Here's how the part is built. I have some questions about the finished solid (model axes, mm). Face numbers are marked on the shaded views. A direction names the side the tool comes from. Give positions to 0.01 mm unless a question says otherwise; leave off trailing zeros. Loops run counter-clockwise (first coordinate to the right, second up) from the corner with the lowest first, then second, coordinate; pieces in that order, holes last.
Q1. For the marked faces 4, 5 and 6, which set-ups out of +Z, -Z, +X, -X, +Y, -Y let a thin tool reach every point of the face, with its end or its side?
Q2. I need wall thicknesses on probe 1 along X at (y, z) = (14.5, 7.5); probe 2 along X at (y, z) = (4, 7); probe 3 along Y at (x, z) = (2, -16.5). Which ranges of each line are inside material? Lowest first, please.
Q3. Suppose I cut it at C-C (y = 13.5). List the corners of the cut face in (x, z) for me, and give its area (3 significant figures).
Q4. Suppose I cut it at B-B (z = 0). List the corners of the cut face in (x, y) for me, and give its area (3 significant figures).
Q5. Suppose I cut it at D-D (y = 6.5). List the corners of the cut face in (x, z) for me.
Q6. Suppose I cut it at A-A (x = 0). List the corners of the cut face in (y, z) for me, and give its area (3 significant figures).
Q7. Thinking about a two-plate mould opening in X: for the marked faces 1, 2 and 3, which applies, pulls with the +X half, pulls with the -X half, needs draft (parallel to the pull), parting line crosses it, or undercut?
Q8. I'm going to push flat-ended pins straight in: P1, Ø2, axis at x = -1, z = 21.5, coming from the -Y side; P2, Ø6.5, axis at x = -12.99, z = 7.5, coming from the -Y side; P3, Ø1, axis at x = 15.5, z = -16, coming from the +Y side; P4, Ø1, axis at x = -15, y = 10, coming from the -Z side. Where does each tip first touch, or does it pass through?
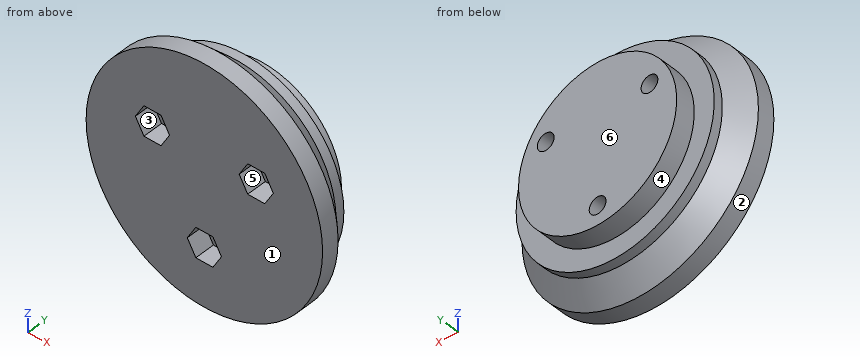
```python
from build123d import *

# Parameters (mm, degrees)
CUT_EXTRUDE1_REACH = 46.995
SKETCH2_R          = 2.1
CUT_EXTRUDE2_DEPTH = 5


with BuildPart() as part:
    # Sketch1 → Revolve1 (revolve)
    with BuildSketch(Plane.XY):
        Polygon((0, 16.5), (19.8, 16.5), (19.8, 11.5), (24.8, 11.5), (24.8, 9.2), (29.6, 4.4), (29.6, 0), (0, 0), align=None)
    revolve(axis=Axis((0, 0, 0), (0, 1, 0)))

    # Sketch2 → Cut-Extrude1 (cut, up to next)
    with BuildSketch(Plane(origin=(0, 16.5, 0), x_dir=(1, 0, 0), z_dir=(0, 1, 0)), mode=Mode.PRIVATE) as cut_extrude1_sk1:
        with Locations(Location((0, 15, 0), (0, 0, 270))):
            Circle(SKETCH2_R)
    cut_extrude1_tool1 = extrude(cut_extrude1_sk1.sketch, amount=-CUT_EXTRUDE1_REACH, mode=Mode.PRIVATE) & part.part
    # Sketch2 → Cut-Extrude1 (cut, up to next)
    with BuildSketch(Plane(origin=(0, 16.5, 0), x_dir=(1, 0, 0), z_dir=(0, 1, 0)), mode=Mode.PRIVATE) as cut_extrude1_sk2:
        with Locations(Location((-12.990381057, -7.5, 0), (0, 0, 270))):
            Circle(SKETCH2_R)
    cut_extrude1_tool2 = extrude(cut_extrude1_sk2.sketch, amount=-CUT_EXTRUDE1_REACH, mode=Mode.PRIVATE) & part.part
    # Sketch2 → Cut-Extrude1 (cut, up to next)
    with BuildSketch(Plane(origin=(0, 16.5, 0), x_dir=(1, 0, 0), z_dir=(0, 1, 0)), mode=Mode.PRIVATE) as cut_extrude1_sk3:
        with Locations(Location((12.990381057, -7.5, 0), (0, 0, 270))):
            Circle(SKETCH2_R)
    cut_extrude1_tool3 = extrude(cut_extrude1_sk3.sketch, amount=-CUT_EXTRUDE1_REACH, mode=Mode.PRIVATE) & part.part
    add(cut_extrude1_tool1.solids().sort_by_distance((0, 16.5, -15))[0], mode=Mode.SUBTRACT)
    add(cut_extrude1_tool2.solids().sort_by_distance((-12.990381, 16.5, 7.5))[0], mode=Mode.SUBTRACT)
    add(cut_extrude1_tool3.solids().sort_by_distance((12.990381, 16.5, 7.5))[0], mode=Mode.SUBTRACT)

    # Sketch3 → Cut-Extrude2 (cut)
    with BuildSketch(Plane.XZ):
        Polygon((-10.854185061, 11.2), (-15.126577053, 11.2), (-17.262773049, 7.5), (-15.126577053, 3.8), (-10.854185061, 3.8), (-8.717989065, 7.5), align=None)
        Polygon((15.126577053, 11.2), (10.854185061, 11.2), (8.717989065, 7.5), (10.854185061, 3.8), (15.126577053, 3.8), (17.262773049, 7.5), align=None)
        Polygon((2.136195996, -11.3), (-2.136195996, -11.3), (-4.272391992, -15), (-2.136195996, -18.7), (2.136195996, -18.7), (4.272391992, -15), align=None)
    extrude(amount=-CUT_EXTRUDE2_DEPTH, mode=Mode.SUBTRACT)


solid = part.part
```
Solutions:
1. face 4: +Y
1. face 5: -Y
1. face 6: +Z, -Z, +X, -X, +Y
2. probe 1: x = -18.32 to -15.09, -10.89 to 10.89, 15.09 to 18.32
2. probe 2: x = -28.76 to -16.97, -9.01 to 9.01, 16.97 to 28.76
2. probe 3: y = 5 to 16.5
3. outline: circle Ø39.6 at (0, 0); hole circle Ø4.2 at (-12.99, 7.5); hole circle Ø4.2 at (0, -15); hole circle Ø4.2 at (12.99, 7.5)
3. area: 1,190 mm2
4. outline: (-29.6, 0) - (29.6, 0) - (29.6, 4.4) - (24.8, 9.2) - (24.8, 11.5) - (19.8, 11.5) - (19.8, 16.5) - (-19.8, 16.5) - (-19.8, 11.5) - (-24.8, 11.5) - (-24.8, 9.2) - (-29.6, 4.4) - close
4. area: 834 mm2
5. outline: circle Ø55 at (0, 0); hole circle Ø4.2 at (-12.99, 7.5); hole circle Ø4.2 at (0, -15); hole circle Ø4.2 at (12.99, 7.5)
6. outline: (0, -29.6) - (4.4, -29.6) - (9.2, -24.8) - (11.5, -24.8) - (11.5, -19.8) - (16.5, -19.8) - (16.5, -17.1) - (5, -17.1) - (5, -18.7) - (0, -18.7) - close; (0, -11.3) - (5, -11.3) - (5, -12.9) - (16.5, -12.9) - (16.5, 19.8) - (11.5, 19.8) - (11.5, 24.8) - (9.2, 24.8) - (4.4, 29.6) - (0, 29.6) - close
6. area: 748 mm2
7. face 1: needs draft
7. face 2: parting line crosses it
7. face 3: undercut
8. P1: stops at y = 0
8. P2: stops at y = 5
8. P3: stops at y = 11.5
8. P4: stops at z = -20.12
